The drawing under review shows one solid part. Ordinate dimensions are in mm from its lowest x, y, z. A direction names the side the tool comes from. Coordinates: 2 decimals unless noted, no trailing zeros. Write each loop counter-clockwise with the first axis right and the second up, starting at its lowest first coordinate (ties: lowest second). Pieces come first, ordered by that corner, then holes.
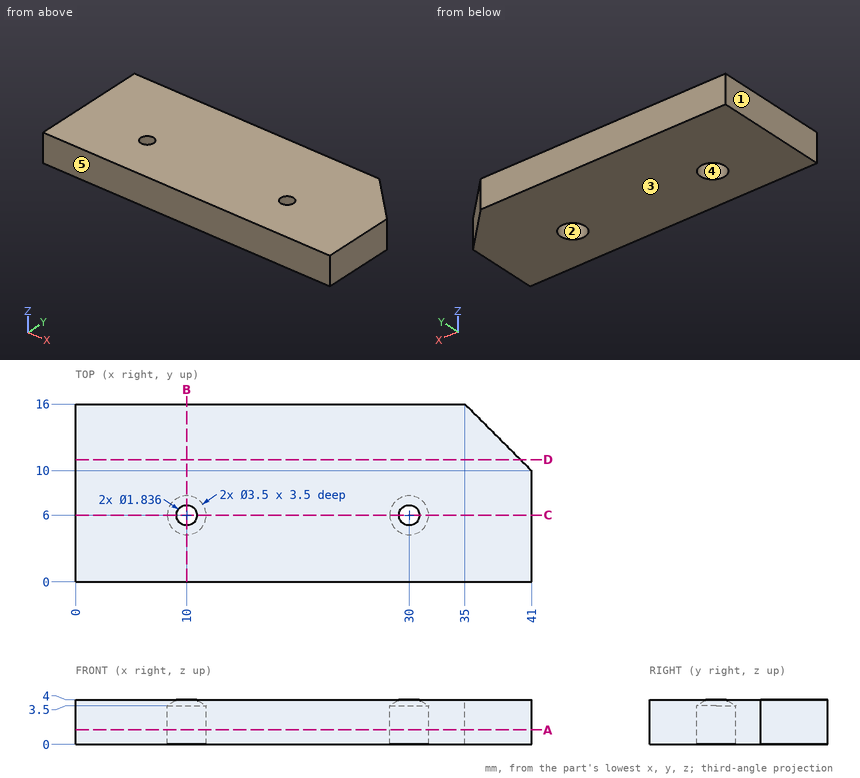
Q1. Add section D-D (y = 11). State the section outline as (x, z) points.
Ans:
outline: (0, 0) - (40, 0) - (40, 4) - (0, 4) - close
Q2. For probe 1 along X at (y, z) = (6, 2.3); probe 2 along Y at (x, z) = (10, 2.3); probe 3 along X at (y, z) = (12, 3.7), list the stretches that pass through material, from the lowest coordinate up.
Ans:
probe 1: x = 0 to 8.25, 11.75 to 28.25, 31.75 to 41
probe 2: y = 0 to 4.25, 7.75 to 16
probe 3: x = 0 to 39
Q3. Draft analysis for pull direction Y (two halves, no side actions). For the marked faces 3, 4 and 5, state which applies: +Y half, -Y half, draft (parallel to the pull), parting line (faces both ways), or undercut.
Ans:
face 3: draft
face 4: undercut
face 5: -Y half
Q4. Add section B-B (x = 10). State the section outline as (y, z) points, then the cut area to 3 significant figures.
Ans:
outline: (0, 0) - (4.25, 0) - (4.25, 3.5) - (5.08, 4) - (0, 4) - close; (6.92, 4) - (7.75, 3.5) - (7.75, 0) - (16, 0) - (16, 4) - close
area: 50.4 mm2
Q5. Add section A-A (z = 1.3). State the section outline as (x, y) points.
Ans:
outline: (0, 0) - (41, 0) - (41, 10) - (35, 16) - (0, 16) - close; hole circle Ø3.5 at (10, 6); hole circle Ø3.5 at (30, 6)
Q6. Add section C-C (y = 6). State the section outline as (x, z) points.
Ans:
outline: (0, 0) - (8.25, 0) - (8.25, 3.5) - (9.08, 4) - (0, 4) - close; (10.92, 4) - (11.75, 3.5) - (11.75, 0) - (28.25, 0) - (28.25, 3.5) - (29.08, 4) - close; (30.92, 4) - (31.75, 3.5) - (31.75, 0) - (41, 0) - (41, 4) - close
Q7. Tool access review of the marked faces 1 and 2: name each direction out of +Z, -Z, +X, -X, +Y, -Y from which nothing blocks a thin tool from reaching the whole face with its end or side.
Ans:
face 1: +Z, -Z, -X, +Y, -Y
face 2: -Z
Q8. Clearance check with a flat-ended pin moving along its axis: pin 1 Ø1 at (y, z) = (11.5, 1) entering from +X. State where the tip first meets the part, or that it passes through.
Ans:
pin 1: stops at x = 40
